Part model, mm, in its own coordinate system. A direction names the side the tool comes from. Give positions to 0.01 mm unless a question says otherwise; leave off trailing zeros. Order: outer loops, then holes, each group sorted by start corner. A loop starts at its lowest first (then second) coordinate and runs counter-clockwise, first axis right, second up. Notation, with made-up numbers: (49, 70) - (64, 70) arc R25 cw to (64, 86) - close; hole circle Ø10 at (-14, 53.5). An arc over 180 degrees is marked (long way). Use one line per item in the form item = value. Start each with the question number.
1. Drill centre lines: line 1 (X direction, y = 19, z = 1.9); line 2 (Z direction, x = -0.1, y = 2). Where is each one in solid material? Low to high.
2. Pin check, flat tips, straight feed: P1, Ø2.5, axis at y = 40, z = -0.5, coming from the +X side; P2, Ø2, axis at y = 32.5, z = -2.5, coming from the +X side; P3, Ø0.5, axis at x = 2.5, z = 0.5, coming from the +Y side. Stop position of each tip, or through.
3. Band-saw the part on B-B, the plane y = 10. List the corners of the cut face in (x, z).
4. Band-saw the part on A-A, the plane z = 0. List the corners of the cut face in (x, y), plus the area to 3 significant figures.
5. Pull direction Z, two halves, no side cores. Call faces 1 (the face through (0, 45, -0.75)), 2 (the face through (-3, 23, 0)), 3 (the face through (0, 0, 0)): +Z half, -Z half, draft (parallel to the pull), parting line (faces both ways), or undercut.
6. Tool access for faces 4 (the face through (-0.854, 45.865, 2.493)), 5 (the face through (1.9, 40, 0)), 6 (the face through (-1, 45, 0.75)): list every direction of +Z, -Z, +X, -X, +Y, -Y with a clear straight run to the whole face (end or side of a thin tool).
from build123d import *

# Parameters (mm, degrees)
SKIZZE1_R                       = 3
AUFSATZ_LINEAR_AUSTRAGEN1_DEPTH = 46
SKIZZE2_W                       = 2.221209883
SKIZZE2_H                       = 8.751437557
SCHNITT_LINEAR_AUSTRAGEN1_DEPTH = 11.5
FASE1_SIZE                      = 0.5
SCHNITT_LINEAR_AUSTRAGEN2_DEPTH = 2


with BuildPart() as part:
    # Skizze1 → Aufsatz-Linear austragen1 (new body)
    with BuildSketch(Plane(origin=(0, 0, 0), x_dir=(1, 0, 0), z_dir=(0, 1, 0))):
        Circle(SKIZZE1_R)
    extrude(amount=AUFSATZ_LINEAR_AUSTRAGEN1_DEPTH)

    # Skizze2 → Schnitt-Linear austragen1 (cut)
    with BuildSketch(Plane(origin=(0, 46, 0), x_dir=(1, 0, 0), z_dir=(0, 1, 0))):
        with Locations((3.010604942, -0.571236499)):
            Rectangle(SKIZZE2_W, SKIZZE2_H)
    extrude(amount=-SCHNITT_LINEAR_AUSTRAGEN1_DEPTH, mode=Mode.SUBTRACT)

    # Fase1
    fase1_edges = [part.edges().sort_by_distance(p)[0] for p in [
        (-3, 0, 0),
        (-3, 46, 0),
        (1.9, 46, 0),
    ]]
    chamfer(fase1_edges, length=FASE1_SIZE)

    # Skizze3 → Schnitt-Linear austragen2 (cut)
    with BuildSketch(Plane(origin=(0, 46, 0), x_dir=(1, 0, 0), z_dir=(0, 1, 0))):
        Polygon((-4.20448111, 0.75), (0.75, 0.75), (4.606648868, 0.75), (4.606648868, -0.75), (0.75, -0.75), (-4.20448111, -0.75), align=None)
    extrude(amount=-SCHNITT_LINEAR_AUSTRAGEN2_DEPTH, mode=Mode.SUBTRACT)


solid = part.part
From the geometry:
q1.line_1 = -2.32 to 2.32
q1.line_2 = -3 to 3
q2.P1 = 1.9
q2.P2 = 2.6
q2.P3 = 34.5
q3.outline = circle Ø6 at (0, 0)
q4.outline = (-3, 0.5) - (-2.5, 0) - (2.5, 0) - (3, 0.5) - (3, 34.5) - (1.9, 34.5) - (1.9, 44) - (-3, 44) - close
q4.area = 253 mm²
q5.face_1 = undercut
q5.face_2 = parting line
q5.face_3 = draft
q6.face_4 = +Z, +Y
q6.face_5 = +Z, -Z, +X, +Y
q6.face_6 = +X, -X, +Y
